The model under review builds one solid part; all positions refer to its coordinate system, in mm. A direction names the side the tool comes from. Coordinates: 2 decimals unless noted, no trailing zeros. Loops run counter-clockwise (first coordinate to the right, second up) from the corner with the lowest first, then second, coordinate; pieces in that order, holes last. Notation, with made-up numbers: M -11.5,65 L 29.5,65 A11 ccw 29.5,84 Z; hole C 85,79 d3. An arc over 180 degrees is marked long. Return JSON: item names as keys, results as strings.
```python
from build123d import *

# Parameters (mm, degrees)
EXTRUDE_1_DEPTH      = 5
EXTRUDE_1_DEPTH_BACK = 5
SKETCH_1_W           = 25
SKETCH_1_H           = 25
SKETCH_8_W           = 25
SKETCH_8_H           = 7
CUT_EXTRUDE_8_DEPTH  = 6
SKETCH_9_W           = 25
SKETCH_9_H           = 7
CUT_EXTRUDE_9_DEPTH  = 6
SKETCH_2_R           = 3.5
CUT_EXTRUDE_1_DEPTH  = 10
SKETCH_4_R           = 1.25
CUT_EXTRUDE_3_DEPTH  = 6
SKETCH_7_R           = 3
CUT_EXTRUDE_7_DEPTH  = 21.910523666


with BuildPart() as part:
    # Sketch 1 → Extrude 1 (new, two sides: drawn at the far end of the back side and taken through both)
    with BuildSketch(Plane(origin=(0, 0, 0), x_dir=(1, 0, 0), z_dir=(0, 1, 0)).offset(-EXTRUDE_1_DEPTH_BACK)):
        Rectangle(SKETCH_1_W, SKETCH_1_H)
    extrude(amount=EXTRUDE_1_DEPTH + EXTRUDE_1_DEPTH_BACK)

    # Sketch 8 → Cut-Extrude 8 (cut)
    with BuildSketch(Plane(origin=(-12.5, 0, 0), x_dir=(0, 0, -1), z_dir=(1, 0, 0))):
        Rectangle(SKETCH_8_W, SKETCH_8_H)
    cut_extrude_8 = extrude(amount=CUT_EXTRUDE_8_DEPTH, mode=Mode.SUBTRACT)

    # Mirror 1: Cut-Extrude 8 across plane
    add(cut_extrude_8.mirror(Plane(origin=(0, 0, 0), x_dir=(0, 0, 1), z_dir=(1, 0, 0))), mode=Mode.SUBTRACT)

    # Sketch 9 → Cut-Extrude 9 (cut)
    with BuildSketch(Plane.XY.offset(12.5)):
        Rectangle(SKETCH_9_W, SKETCH_9_H)
    cut_extrude_9 = extrude(amount=-CUT_EXTRUDE_9_DEPTH, mode=Mode.SUBTRACT)

    # Mirror 2: Cut-Extrude 9 across plane
    add(cut_extrude_9.mirror(Plane.XY), mode=Mode.SUBTRACT)

    # Sketch 2 → Cut-Extrude 1 (cut)
    with BuildSketch(Plane(origin=(-6.5, 0, 0), x_dir=(0, 0, -1), z_dir=(1, 0, 0))):
        with Locations(Location((1, 0, 0), (0, 0, 90))):
            Circle(SKETCH_2_R)
    extrude(amount=CUT_EXTRUDE_1_DEPTH, mode=Mode.SUBTRACT)

    # Sketch 4 → Cut-Extrude 3 (cut)
    with BuildSketch(Plane(origin=(-6.5, 0, 0), x_dir=(0, 0, -1), z_dir=(1, 0, 0))):
        with Locations((-3.3, 0)):
            Circle(SKETCH_4_R)
    extrude(amount=CUT_EXTRUDE_3_DEPTH, mode=Mode.SUBTRACT)

    # Sketch 7 → Cut-Extrude 7 (cut, through all)
    with BuildSketch(Plane.ZY.offset(-3.5)):
        with Locations((-1, 0)):
            Circle(SKETCH_7_R)
    extrude(amount=-CUT_EXTRUDE_7_DEPTH, mode=Mode.SUBTRACT)


solid = part.part
```
1. Add section A-A on z = 10. Give the boundary of the cut face in (x, y).
Check values:
{"outline": "M -12.5,-5 L 12.5,-5 L 12.5,-3.5 L -12.5,-3.5 Z; M -12.5,3.5 L 12.5,3.5 L 12.5,5 L -12.5,5 Z"}
2. Insertion check: pin 1 Ø4 at (y, z) = (0, 3.3) entering from -X; pin 2 Ø3 at (y, z) = (1.5, -0.5) entering from -X; pin 3 Ø5.5 at (x, y) = (-2.5, -1.5) entering from +Z; pin 4 Ø1.5 at (y, z) = (1.5, 6.5) entering from +X. Each pin has a flat end and moves straight along its axis. Give the tip position at first contact, or say it passes through.
Check values:
{"pin 1": "x = -6.5", "pin 2": "x = 3.5", "pin 3": "z = 12.5", "pin 4": "x = 6.5"}
3. Add section B-B on x = 7.75. Give the boundary of the cut face in (y, z), plus the area to 3 significant figures.
Check values:
{"outline": "M -5,-12.5 L -3.5,-12.5 L -3.5,12.5 L -5,12.5 Z; M 3.5,-12.5 L 5,-12.5 L 5,12.5 L 3.5,12.5 Z", "area": "75.0 mm²"}
4. The part is to be moulded in two halves that separate along Z. For faces 5 (the face through (0, 4, -12.5)), 6 (the face through (3.5, 3, 0)), 7 (the face through (-3.54, 0.04, 4.55)), 8 (the face through (0, 4, 12.5)), say which applies: released by +Z, released by -Z, zero draft, split by the parting line, or undercut.
Check values:
{"face 5": "released by -Z", "face 6": "undercut", "face 7": "undercut", "face 8": "released by +Z"}
5. Add section D-D on y = 0. Give the boundary of the cut face in (x, z).
Check values:
{"outline": "M -6.5,-6.5 L 6.5,-6.5 L 6.5,-4 L 3.5,-4 L 3.5,-4.5 L -6.5,-4.5 Z; M -6.5,4.55 L -0.5,4.55 L -0.5,2.5 L 3.5,2.5 L 3.5,2 L 6.5,2 L 6.5,6.5 L -6.5,6.5 Z"}
6. To check wall thickness, follow line 1 (Z direction, x = -4, y = 0); line 2 (Y direction, x = 8.25, z = 10); line 3 (Y direction, x = -2.6, z = 3.3). State the ranges of each line that lie inside material, in increasing order.
Check values:
{"line 1": "-6.5 to -4.5, 4.55 to 6.5", "line 2": "-5 to -3.5, 3.5 to 5", "line 3": "-5 to -1.25, 1.25 to 5"}
7. Add section C-C on x = 1.25. Give the boundary of the cut face in (y, z), plus the area to 3 significant figures.
Check values:
{"outline": "M -5,-12.5 L -3.5,-12.5 L -3.5,-6.5 L 3.5,-6.5 L 3.5,-12.5 L 5,-12.5 L 5,12.5 L 3.5,12.5 L 3.5,6.5 L -3.5,6.5 L -3.5,12.5 L -5,12.5 Z; hole C 0,-1 d7", "area": "128 mm²"}
8. Machinability: for faces 1 (the face through (0, 0, 6.5)), 2 (the face through (0, 3.5, 9)), 3 (the face through (6.5, 2, 2)), 4 (the face through (0, 0, -6.5)), which of the approach directions +Z, -Z, +X, -X, +Y, -Y give a long, thin tool a straight path to every point of the face, cutting with its end or side? Answer none if there is none.
Check values:
{"face 1": "+Z, +X, -X", "face 2": "none", "face 3": "+Z, -Z, +X", "face 4": "-Z, +X, -X"}
